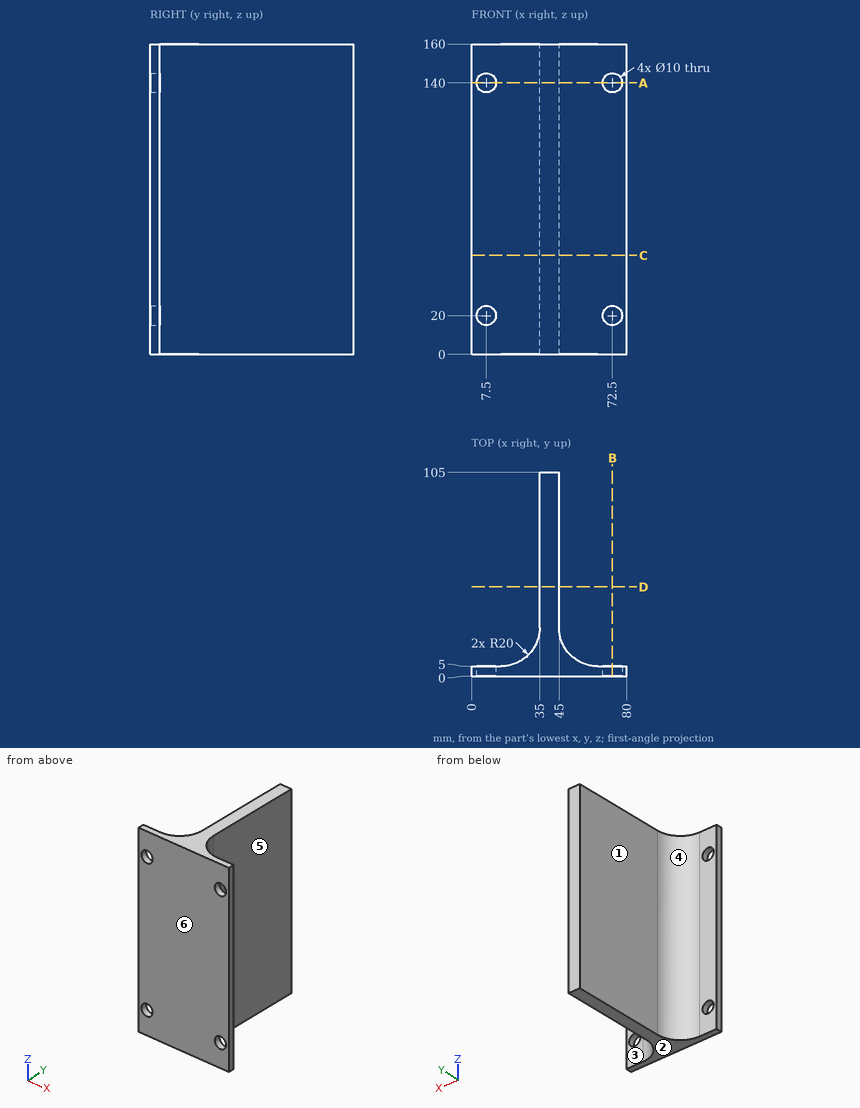
Job drawing, mm, ordinate dimensions from the low corner. One solid piece. A direction names the side the tool comes from. Round coordinates to 2 decimals unless told otherwise and drop trailing zeros. Order: outer loops, then holes, each group sorted by start corner. A loop starts at its lowest first (then second) coordinate and runs counter-clockwise, first axis right, second up. Notation, with made-up numbers: (24, -8) -> (41, -8) arc R18 cw to (41, -1) -> close; hole circle Ø7 at (89.5, 8.25). An arc over 180 degrees is marked (long way). Write item = value, one per line.
(1) Pull direction Y, two halves, no side cores. Call the marked faces 4, 5 and 6: +Y half, -Y half, draft (parallel to the pull), parting line (faces both ways), or undercut.
Answers follow:
face_4 = +Y half
face_5 = draft
face_6 = -Y half
(2) Flat gauge pins, fed straight in: P1, Ø9, axis at x = 72.5, z = 20, coming from the +Y side; P2, Ø13, axis at x = 7.5, z = 20, coming from the +Y side; P3, Ø1.5, axis at x = 59, z = 50.5, coming from the +Y side; P4, Ø2, axis at y = 87.5, z = 71, coming from the -X side. Where does each tip first touch, or does it go through?
Answers follow:
P1 = through
P2 = 5
P3 = 6.17
P4 = 35
(3) Cut at C-C (z = 51). Write the cut outline in (x, y).
Answers follow:
outline = (0, 0) -> (80, 0) -> (80, 5) -> (65, 5) arc R20 cw to (45, 25) -> (45, 105) -> (35, 105) -> (35, 25) arc R20 cw to (15, 5) -> (0, 5) -> close
(4) Cut at A-A (z = 140). Write the cut outline in (x, y), plus the area to 3 significant figures.
Answers follow:
outline = (0, 0) -> (2.5, 0) -> (2.5, 5) -> (0, 5) -> close; (12.5, 0) -> (67.5, 0) -> (67.5, 5) -> (65, 5) arc R20 cw to (45, 25) -> (45, 105) -> (35, 105) -> (35, 25) arc R20 cw to (15, 5) -> (12.5, 5) -> close; (77.5, 0) -> (80, 0) -> (80, 5) -> (77.5, 5) -> close
area = 1,470 mm²
(5) Cut at D-D (y = 46). Write the cut outline in (x, z), plus the area to 3 significant figures.
Answers follow:
outline = (35, 0) -> (45, 0) -> (45, 160) -> (35, 160) -> close
area = 1,600 mm²
(6) 3-axis set-ups, long thin cutter, end or side, ignore diameter. For the marked faces 1, 2 and 3: which of +Z, -Z, +X, -X, +Y, -Y reach the whole face in a straight line?
Answers follow:
face_1 = +Z, -Z, -X, +Y
face_2 = -Z, +X, -X, +Y, -Y
face_3 = +Z, -Z, +X, +Y
(7) Drill centre lines: L1, parallel to Z at x = 72.5, y = 1.4; L2, parallel to X at y = 2, z = 20; L3, parallel to X at y = 74, z = 149. Where is each one in solid material? Low to high.
Answers follow:
L1 = 0 to 15, 25 to 135, 145 to 160
L2 = 0 to 2.5, 12.5 to 67.5, 77.5 to 80
L3 = 35 to 45
(8) Cut at B-B (x = 72.5). Write the cut outline in (y, z).
Answers follow:
outline = (0, 0) -> (5, 0) -> (5, 15) -> (0, 15) -> close; (0, 25) -> (5, 25) -> (5, 135) -> (0, 135) -> close; (0, 145) -> (5, 145) -> (5, 160) -> (0, 160) -> close
